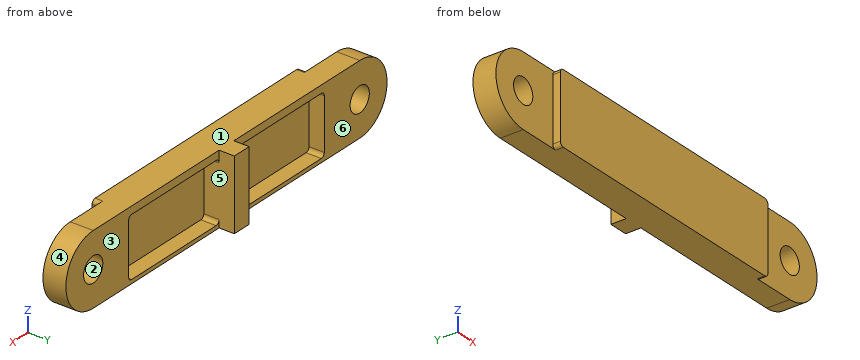
from build123d import *

# Parameters (mm, degrees)
SKETCH1_W           = 35.1
SKETCH1_H           = 18.5
BOSS_EXTRUDE1_DEPTH = 8
SKETCH10_R          = 3.25
BOLT_EXTRUDE_DEPTH  = 6
SKETCH7_W           = 33.1
SKETCH7_H           = 15.5
CUT_EXTRUDE5_DEPTH  = 4
SKETCH8_W           = 5
SKETCH8_H           = 18.5
BOSS_EXTRUDE3_DEPTH = 8
FILLET6_R           = 1


with BuildPart() as part:
    # Sketch1 → Boss-Extrude1 (new body)
    with BuildSketch(Plane(origin=(0, 0, 0), x_dir=(1, 0, 0), z_dir=(0, 1, 0))):
        with Locations((-17.55, 0)):
            Rectangle(SKETCH1_W, SKETCH1_H)
    extrude(amount=BOSS_EXTRUDE1_DEPTH)

    # Sketch10 → bolt extrude (add)
    with BuildSketch(Plane(origin=(0, 8, 0), x_dir=(1, 0, 0), z_dir=(0, 1, 0))):
        with BuildLine():
            Line((-35.1, 9.25), (-45.1, 9.25))
            ThreePointArc((-45.1, 9.25), (-54.35, 0), (-45.1, -9.25))
            Line((-45.1, -9.25), (-35.1, -9.25))
            Line((-35.1, -9.25), (-35.1, 9.25))
        make_face()
        with Locations(Location((-45.1, 0, 0), (0, 0, 270))):
            Circle(SKETCH10_R, mode=Mode.SUBTRACT)
    extrude(amount=-BOLT_EXTRUDE_DEPTH)

    # Sketch7 → Cut-Extrude5 (cut)
    with BuildSketch(Plane(origin=(0, 8, 0), x_dir=(1, 0, 0), z_dir=(0, 1, 0))):
        with Locations((-16.55, 0.5)):
            Rectangle(SKETCH7_W, SKETCH7_H)
    extrude(amount=-CUT_EXTRUDE5_DEPTH, mode=Mode.SUBTRACT)

    # Mirror1: part across plane


with BuildPart() as part_1:
    add(part.part)
    add(part.part.mirror(Plane(origin=(0, 0, 0), x_dir=(0, 0, 1), z_dir=(1, 0, 0))))

    # Sketch8 → Boss-Extrude3 (add)
    with BuildSketch(Plane(origin=(0, 4, 0), x_dir=(1, 0, 0), z_dir=(0, 1, 0))):
        Rectangle(SKETCH8_W, SKETCH8_H)
    extrude(amount=BOSS_EXTRUDE3_DEPTH)

    # Fillet6
    fillet6_edges = [part_1.edges().sort_by_distance(p)[0] for p in [
        (-35.1, 1, 9.25),
        (-35.1, 1, -9.25),
        (-33.1, 6, -8.25),
        (-33.1, 6, 7.25),
        (35.1, 1, -9.25),
        (35.1, 1, 9.25),
        (33.1, 6, -8.25),
        (33.1, 6, 7.25),
        (-2.5, 6, 7.25),
        (2.5, 6, 7.25),
        (2.5, 6, -8.25),
        (-2.5, 6, -8.25),
    ]]
    fillet(fillet6_edges, radius=FILLET6_R)


solid = part_1.part
Geometry check sheet. Reference: the model listing, model coordinates, mm. Face numbers are marked on the shaded views. A direction names the side the tool comes from. Give positions to 0.01 mm unless a question says otherwise; leave off trailing zeros. Write each loop counter-clockwise with the first axis right and the second up, starting at its lowest first coordinate (ties: lowest second). Pieces come first, ordered by that corner, then holes.
1) Set-up check for the marked faces 4, 5 and 6: record each of +Z, -Z, +X, -X, +Y, -Y from which the full face is reachable in a straight line by a thin tool's end or side.
Values follow:
face 4: +X, +Y, -Y
face 5: +Y
face 6: +Z, -Z, -X, +Y
2) Release check for a two-part mould opening along Z. For the marked faces 1, 2 and 3 record: released by +Z, released by -Z, zero draft, split by the parting line, or undercut.
Values follow:
face 1: released by +Z
face 2: undercut
face 3: zero draft
3) Go/stop test with flat-tipped pins: pin 1 Ø3 at (y, z) = (6, -7.5) entering from -X; pin 2 Ø10.5 at (x, z) = (-45.1, 0) entering from +Y; pin 3 Ø2 at (y, z) = (1.5, -4.5) entering from -X. Record where each tip stops, or that it passes through.
Values follow:
pin 1: stops at x = -52.14
pin 2: stops at y = 8
pin 3: stops at x = -53.61
4) Cross-section at B-B (x = -43). Record the boundary of the cut face in (y, z), plus the area to 3 significant figures.
Values follow:
outline: (2, -9.25) - (8, -9.25) - (8, -2.48) - (2, -2.48) - close; (2, 2.48) - (8, 2.48) - (8, 9.25) - (2, 9.25) - close
area: 81.2 mm2
5) Cross-section at C-C (x = -14). Record the boundary of the cut face in (y, z).
Values follow:
outline: (0, -9.25) - (8, -9.25) - (8, -8.25) - (4, -8.25) - (4, 7.25) - (8, 7.25) - (8, 9.25) - (0, 9.25) - close
6) Thickness scan on line 1 (X direction, y = 3.3, z = 0); line 2 (X direction, y = 4.9, z = 0); line 3 (X direction, y = 4.75, z = 3.5). Record the ranges inside material, lowest first.
Values follow:
line 1: x = -54.35 to -48.35, -41.85 to 41.85, 48.35 to 54.35
line 2: x = -54.35 to -48.35, -41.85 to -33.1, -2.5 to 2.5, 33.1 to 41.85, 48.35 to 54.35
line 3: x = -53.66 to -33.1, -2.5 to 2.5, 33.1 to 53.66
7) Cross-section at D-D (z = -5.75). Record the boundary of the cut face in (x, y).
Values follow:
outline: (-52.35, 2) - (-35.1, 2) - (-35.1, 0) - (35.1, 0) - (35.1, 2) - (52.35, 2) - (52.35, 8) - (33.1, 8) - (33.1, 4) - (2.5, 4) - (2.5, 12) - (-2.5, 12) - (-2.5, 4) - (-33.1, 4) - (-33.1, 8) - (-52.35, 8) - close
8) Cross-section at A-A (z = 0). Record the boundary of the cut face in (x, y).
Values follow:
outline: (-54.35, 2) - (-48.35, 2) - (-48.35, 8) - (-54.35, 8) - close; (-41.85, 2) - (-35.1, 2) - (-35.1, 0) - (35.1, 0) - (35.1, 2) - (41.85, 2) - (41.85, 8) - (33.1, 8) - (33.1, 4) - (2.5, 4) - (2.5, 12) - (-2.5, 12) - (-2.5, 4) - (-33.1, 4) - (-33.1, 8) - (-41.85, 8) - close; (48.35, 2) - (54.35, 2) - (54.35, 8) - (48.35, 8) - close
